Read the model definition and answer for the solid it produces. Units are mm, in the model's axes. Coordinates: 2 decimals unless noted, no trailing zeros. Order: outer loops, then holes, each group sorted by start corner. A loop starts at its lowest first (then second) coordinate and runs counter-clockwise, first axis right, second up. Notation, with made-up numbers: (67, 69) -> (97, 69) arc R21 cw to (97, 79) -> close; hole circle Ø4 at (68, 2). An arc over 180 degrees is marked (long way). Use CSV: the item, a comma, the result in double quotes.
```python
from build123d import *

# Parameters (mm, degrees)
F0_W     = 25
F0_H     = 25
F1_DEPTH = 240


with BuildPart() as f1:
    # F0 (on Front) → F1 (new body)
    with BuildSketch(Plane.XZ):
        with BuildLine():
            Line((-37.5, -45.5), (-37.5, -57.5))
            Line((-37.5, -57.5), (37.5, -57.5))
            Line((37.5, -57.5), (37.5, -45.5))
            ThreePointArc((37.5, -45.5), (38.232233, -43.732233), (40, -43))
            Line((40, -43), (40, -41))
            ThreePointArc((40, -41), (37.5, -38.5), (40, -36))
            Line((40, -36), (40, -34))
            ThreePointArc((40, -34), (37.5, -31.5), (40, -29))
            Line((40, -29), (40, -27))
            ThreePointArc((40, -27), (37.5, -24.5), (40, -22))
            Line((40, -22), (40, -20))
            ThreePointArc((40, -20), (37.5, -17.5), (40, -15))
            Line((40, -15), (40, -13))
            ThreePointArc((40, -13), (37.5, -10.5), (40, -8))
            Line((40, -8), (40, -6))
            ThreePointArc((40, -6), (37.5, -3.5), (40, -1))
            Line((40, -1), (40, 1))
            ThreePointArc((40, 1), (37.5, 3.5), (40, 6))
            Line((40, 6), (40, 8))
            ThreePointArc((40, 8), (37.5, 10.5), (40, 13))
            Line((40, 13), (40, 15))
            ThreePointArc((40, 15), (37.5, 17.5), (40, 20))
            Line((40, 20), (40, 22))
            ThreePointArc((40, 22), (37.5, 24.5), (40, 27))
            Line((40, 27), (40, 29))
            ThreePointArc((40, 29), (37.5, 31.5), (40, 34))
            Line((40, 34), (40, 36))
            ThreePointArc((40, 36), (37.5, 38.5), (40, 41))
            Line((40, 41), (40, 43))
            ThreePointArc((40, 43), (37.5, 45.5), (40, 48))
            Line((40, 48), (40, 57.5))
            Line((40, 57.5), (30.5, 57.5))
            ThreePointArc((30.5, 57.5), (28, 55), (25.5, 57.5))
            Line((25.5, 57.5), (23.5, 57.5))
            ThreePointArc((23.5, 57.5), (21, 55), (18.5, 57.5))
            Line((18.5, 57.5), (16.5, 57.5))
            ThreePointArc((16.5, 57.5), (14, 55), (11.5, 57.5))
            Line((11.5, 57.5), (9.5, 57.5))
            ThreePointArc((9.5, 57.5), (7, 55), (4.5, 57.5))
            Line((4.5, 57.5), (2.5, 57.5))
            ThreePointArc((2.5, 57.5), (0, 55), (-2.5, 57.5))
            Line((-2.5, 57.5), (-4.5, 57.5))
            ThreePointArc((-4.5, 57.5), (-7, 55), (-9.5, 57.5))
            Line((-9.5, 57.5), (-11.5, 57.5))
            ThreePointArc((-11.5, 57.5), (-14, 55), (-16.5, 57.5))
            Line((-16.5, 57.5), (-18.5, 57.5))
            ThreePointArc((-18.5, 57.5), (-21, 55), (-23.5, 57.5))
            Line((-23.5, 57.5), (-25.5, 57.5))
            ThreePointArc((-25.5, 57.5), (-28, 55), (-30.5, 57.5))
            Line((-30.5, 57.5), (-40, 57.5))
            Line((-40, 57.5), (-40, 48))
            ThreePointArc((-40, 48), (-37.5, 45.5), (-40, 43))
            Line((-40, 43), (-40, 41))
            ThreePointArc((-40, 41), (-37.5, 38.5), (-40, 36))
            Line((-40, 36), (-40, 34))
            ThreePointArc((-40, 34), (-37.5, 31.5), (-40, 29))
            Line((-40, 29), (-40, 27))
            ThreePointArc((-40, 27), (-37.5, 24.5), (-40, 22))
            Line((-40, 22), (-40, 20))
            ThreePointArc((-40, 20), (-37.5, 17.5), (-40, 15))
            Line((-40, 15), (-40, 13))
            ThreePointArc((-40, 13), (-37.5, 10.5), (-40, 8))
            Line((-40, 8), (-40, 6))
            ThreePointArc((-40, 6), (-37.5, 3.5), (-40, 1))
            Line((-40, 1), (-40, -1))
            ThreePointArc((-40, -1), (-37.5, -3.5), (-40, -6))
            Line((-40, -6), (-40, -8))
            ThreePointArc((-40, -8), (-37.5, -10.5), (-40, -13))
            Line((-40, -13), (-40, -15))
            ThreePointArc((-40, -15), (-37.5, -17.5), (-40, -20))
            Line((-40, -20), (-40, -22))
            ThreePointArc((-40, -22), (-37.5, -24.5), (-40, -27))
            Line((-40, -27), (-40, -29))
            ThreePointArc((-40, -29), (-37.5, -31.5), (-40, -34))
            Line((-40, -34), (-40, -36))
            ThreePointArc((-40, -36), (-37.5, -38.5), (-40, -41))
            Line((-40, -41), (-40, -43))
            ThreePointArc((-40, -43), (-38.232233, -43.732233), (-37.5, -45.5))
        make_face()
        with Locations((-17.5, -35)):
            Rectangle(F0_W, F0_H, mode=Mode.SUBTRACT)
        with Locations((17.5, -35)):
            Rectangle(F0_W, F0_H, mode=Mode.SUBTRACT)
        with Locations((-17.5, 0)):
            Rectangle(F0_W, F0_H, mode=Mode.SUBTRACT)
        with Locations((-17.5, 35)):
            Rectangle(F0_W, F0_H, mode=Mode.SUBTRACT)
        with Locations((17.5, 0)):
            Rectangle(F0_W, F0_H, mode=Mode.SUBTRACT)
        with Locations((17.5, 35)):
            Rectangle(F0_W, F0_H, mode=Mode.SUBTRACT)
    extrude(amount=F1_DEPTH)


solid = f1.part
```
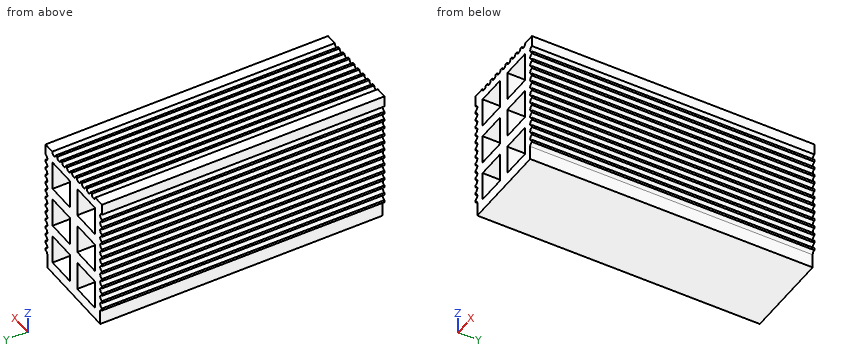
Item 1: Find section C-C, the plane y = -41.5. Give the number of separate pieces and of enclosed holes in the cut face, then the cut area to 3 significant figures.
Return value:
separate pieces,"1"
enclosed holes,"6"
area,"5,040 mm^2"
Item 2: Straight lines are drawn through the part: line 1 along Z through (x, y) = (-17.5, -40.5); line 2 along Z through (x, y) = (-5.5, -221); line 3 along X through (y, z) = (-13.5, -28). For each, find the intervals that lie inside material, in ascending order.
Return value:
line 1,"z = -57.5 to -47.5, -22.5 to -12.5, 12.5 to 22.5, 47.5 to 57.5"
line 2,"z = -57.5 to -47.5, -22.5 to -12.5, 12.5 to 22.5, 47.5 to 55.5"
line 3,"x = -40 to -30, -5 to 5, 30 to 40"
Item 3: Find section B-B, the plane z = -38.5. Give the vertices of the cut face in (x, y).
Return value:
outline,"(-37.5, -240) -> (-30, -240) -> (-30, 0) -> (-37.5, 0) -> close; (-5, -240) -> (5, -240) -> (5, 0) -> (-5, 0) -> close; (30, -240) -> (37.5, -240) -> (37.5, 0) -> (30, 0) -> close"
Item 4: Find section A-A, the plane x = 21. Give the vertices of the cut face in (y, z), then the cut area to 3 significant figures.
Return value:
outline,"(-240, -57.5) -> (0, -57.5) -> (0, -47.5) -> (-240, -47.5) -> close; (-240, -22.5) -> (0, -22.5) -> (0, -12.5) -> (-240, -12.5) -> close; (-240, 12.5) -> (0, 12.5) -> (0, 22.5) -> (-240, 22.5) -> close; (-240, 47.5) -> (0, 47.5) -> (0, 55) -> (-240, 55) -> close"
area,"9,000 mm^2"
Item 5: Each of these flat-tipped pins is pushed along its axis until it touches: P1, Ø13, axis at y = -85, z = -52.5, coming from the -X side; P2, Ø9.5, axis at y = -78, z = -51, coming from the +X side. Where does it stop, or does it pass through?
Return value:
P1,"stops at x = -37.5"
P2,"stops at x = 37.5"
Item 6: Find section D-D, the plane z = -17.5. Give the vertices of the cut face in (x, y).
Return value:
outline,"(-37.5, -240) -> (37.5, -240) -> (37.5, 0) -> (-37.5, 0) -> close"
